```python
from build123d import *

# Parameters (mm, degrees)
CROQUIS1_R              = 12.5
CROQUIS1_R_2            = 7.5
SALIENTE_EXTRUIR1_DEPTH = 38
CROQUIS2_R              = 2.5
SALIENTE_EXTRUIR2_DEPTH = 16.5
CROQUIS3_R              = 7.5
CORTAR_EXTRUIR1_DEPTH   = 38
CROQUIS4_R              = 1.5
SALIENTE_EXTRUIR7_DEPTH = 5
CROQUIS5_R              = 0.5
CORTAR_EXTRUIR2_DEPTH   = 22
ESCALA1_SCALE           = 7


with BuildPart() as part:
    # Croquis1 → Saliente-Extruir1 (new body)
    with BuildSketch(Plane(origin=(0, 0, 0), x_dir=(1, 0, 0), z_dir=(0, 1, 0))):
        Circle(CROQUIS1_R)
        Circle(CROQUIS1_R_2, mode=Mode.SUBTRACT)
    extrude(amount=SALIENTE_EXTRUIR1_DEPTH)

    # Croquis2 → Saliente-Extruir2 (add)
    with BuildSketch(Plane(origin=(0, 0, 0), x_dir=(0, 0, -1), z_dir=(1, 0, 0))):
        with Locations((-2.905741876, 19.965132916)):
            Circle(CROQUIS2_R)
    extrude(amount=SALIENTE_EXTRUIR2_DEPTH)

    # Croquis3 → Cortar-Extruir1 (cut)
    with BuildSketch(Plane(origin=(0, 38, 0), x_dir=(1, 0, 0), z_dir=(0, 1, 0))):
        Circle(CROQUIS3_R)
    extrude(amount=-CORTAR_EXTRUIR1_DEPTH, mode=Mode.SUBTRACT)

    # Croquis4 → Saliente-Extruir7 (add)
    with BuildSketch(Plane(origin=(16.5, 0, 0), x_dir=(0, 0, -1), z_dir=(1, 0, 0))):
        with Locations((-2.933411735, 20.021455872)):
            Circle(CROQUIS4_R)
    extrude(amount=SALIENTE_EXTRUIR7_DEPTH)

    # Croquis5 → Cortar-Extruir2 (cut)
    with BuildSketch(Plane(origin=(21.5, 0, 0), x_dir=(0, 0, -1), z_dir=(1, 0, 0))):
        with Locations((-2.933411735, 20.021455872)):
            Circle(CROQUIS5_R)
    extrude(amount=-CORTAR_EXTRUIR2_DEPTH, mode=Mode.SUBTRACT)


with BuildPart() as part_1:
    # Escala1: scaled about (0.144888953, 19.008953835, 0.027312828)
    add(part.part.scale(ESCALA1_SCALE).moved(Location((-0.869333718, -114.05372301, -0.163876968))))


solid = part_1.part
```
Source: CAD feature listing. Evaluate the final solid. Frame: model axes, mm. A direction names the side the tool comes from. Coordinates: 2 decimals unless noted, no trailing zeros. Loops run counter-clockwise (first coordinate to the right, second up) from the corner with the lowest first, then second, coordinate; pieces in that order, holes last. Notation, with made-up numbers: (-19.75, 24.5) -> (15.25, 24.5) arc R25 ccw to (15.25, 36.5) -> close; hole circle Ø6 at (39.5, 81.5). An arc over 180 degrees is marked (long way). One line per item, written item: value. Start each with the question number.
Q1. Section query B-B, the plane z = -18.5. Return the cut outline in (x, y), and give its area (3 significant figures).
Q2. Section query D-D, the plane y = 12. Return the cut outline in (x, z).
Q3. Line query: line 1 along Z through (x, y) = (0, 99); line 2 along Z through (x, y) = (1.5, 134.5); line 3 along X through (y, z) = (95.5, 1.5). Output: solid intervals per line, ascending.
Q4. Contact query for flat-ended pins moving along their axis: P1, Ø1, axis at y = 74.5, z = 48, coming from the +X side; P2, Ø6, axis at y = -15.5, z = 46.5, coming from the +X side; P3, Ø1, axis at y = -4.5, z = 46, coming from the +X side; P4, Ø17.5, axis at y = 28, z = 23, coming from the +X side. Output: stop coordinate, or through.
Q5. Set-up query: faces 1 (the face through (149.631, 29, 23)), 2 (the face through (131.886, 15.846, 22.646)). Return all of +Z, -Z, +X, -X, +Y, -Y with unobstructed straight access to the full face (end or side cutting, diameter ignored); none if empty.
Q6. Section query A-A, the plane x = -45. Return the cut outline in (y, z).
Q7. Section query C-C, the plane x = 81.5. Return the cut outline in (y, z).
Results:
1. outline: (-86.43, -114.05) -> (-50.06, -114.05) -> (-50.06, 151.95) -> (-86.43, 151.95) -> close; (48.32, -114.05) -> (84.69, -114.05) -> (84.69, 151.95) -> (48.32, 151.95) -> close
1. area: 19,300 mm^2
2. outline: (80.87, 31.06) arc R87.5 ccw (long way) to (86.12, 9.29) -> (114.63, 9.29) -> (114.63, 31.06) -> close; hole circle Ø105 at (-0.87, -0.16)
3. line 1: -87.66 to -52.66, 52.33 to 87.33
3. line 2: -87.63 to -52.61, 52.28 to 87.3
3. line 3: -88.35 to -53.34, 51.6 to 86.61
4. P1: x = 72.51
4. P2: x = 74.96
4. P3: x = 73.77
4. P4: x = 149.63
5. face 1: +Z, -Z, +X, +Y, -Y
5. face 2: +X
6. outline: (-114.05, -75.72) -> (151.95, -75.72) -> (151.95, -28.6) -> (-114.05, -28.6) -> close; (-114.05, 28.27) -> (151.95, 28.27) -> (151.95, 75.39) -> (-114.05, 75.39) -> close
7. outline: (-114.05, -29.69) -> (151.95, -29.69) -> (151.95, 29.36) -> (40.6, 29.36) arc R17.5 ccw to (10.8, 29.36) -> (-114.05, 29.36) -> close; hole circle Ø7 at (26.1, 20.37)
